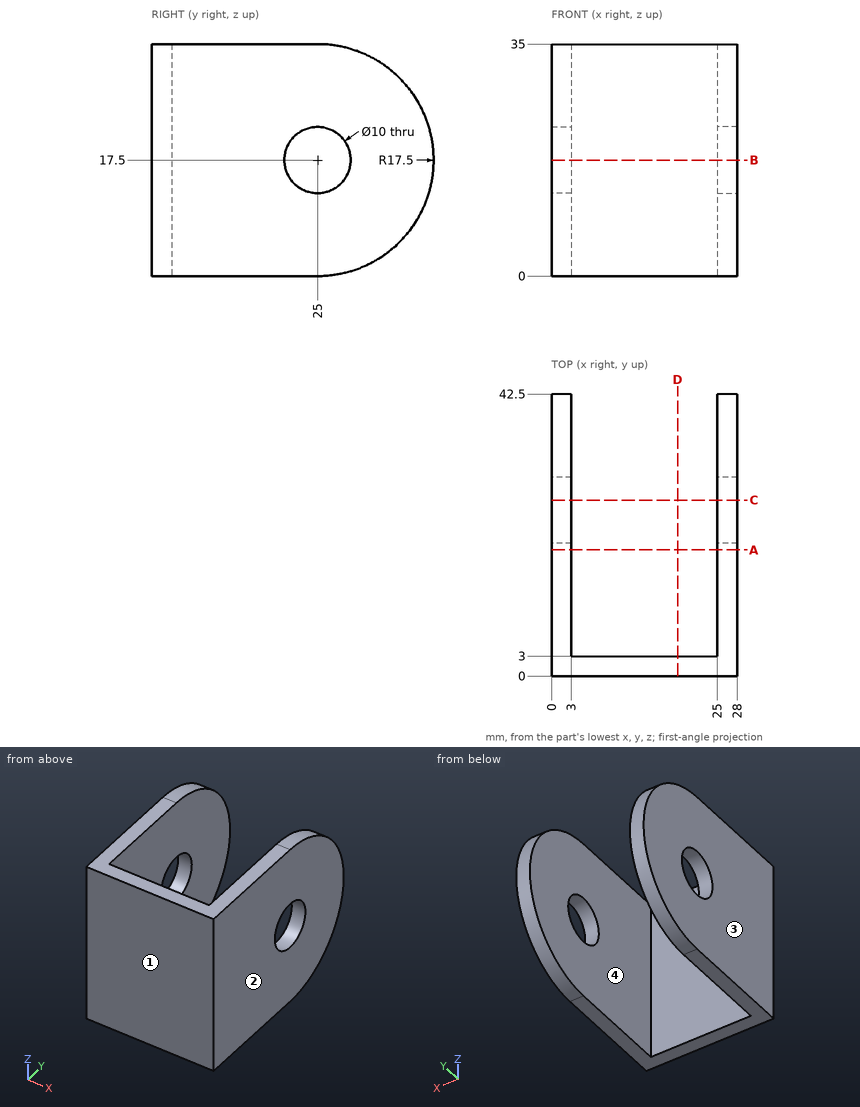
Job drawing, mm, ordinate dimensions from the low corner. One solid piece. Coordinates: 2 decimals unless noted, no trailing zeros. Order: outer loops, then holes, each group sorted by start corner. A loop starts at its lowest first (then second) coordinate and runs counter-clockwise, first axis right, second up. Notation, with made-up numbers: (-13.75, -4.5) -> (34.25, -4.5) arc R8 cw to (34.25, 0.5) -> close; hole circle Ø5 at (-17.75, -31). An arc over 180 degrees is marked (long way). Return JSON: item names as keys, results as strings. Group by question number.
Item 1: Pull direction X, two halves, no side cores. Call the marked faces 1, 2, 3 and 4: pulls with the +X half, pulls with the -X half, needs draft (parallel to the pull), parting line crosses it, or undercut.
Item 2: Wall check: line 1 along X through (y, z) = (31, 33); line 2 along Y through (x, z) = (2.2, 17.5); line 3 along Z through (x, y) = (1.9, 25). Give the ranges that are in metal, low to high. Write a range as [from, to].
Item 3: Saw through at A-A on y = 19. Write the cut outline in (x, z), then the cut area to 3 significant figures.
Item 4: Flat gauge pins, fed straight in: P1, Ø5, axis at x = 10, z = 18.5, coming from the -Y side; P2, Ø11, axis at x = 16.5, z = 17.5, coming from the +Y side. Where does each tip first touch, or does it go through?
Item 5: Saw through at D-D on x = 19. Write the cut outline in (y, z).
Item 6: Saw through at B-B on z = 17.5. Write the cut outline in (x, y).
Item 7: Saw through at C-C on y = 26.5. Write the cut outline in (x, z).
Values found:
{
 "1": {"face 1": "needs draft", "face 2": "pulls with the +X half", "face 3": "pulls with the -X half", "face 4": "undercut"},
 "2": {"line 1": "x = [0, 3], [25, 28]", "line 2": "y = [0, 20], [30, 42.5]", "line 3": "z = [0, 12.5], [22.5, 35]"},
 "3": {"outline": "(0, 0) -> (3, 0) -> (3, 35) -> (0, 35) -> close; (25, 0) -> (28, 0) -> (28, 35) -> (25, 35) -> close", "area": "210 mm2"},
 "4": {"P1": "stops at y = 0", "P2": "stops at y = 3"},
 "5": {"outline": "(0, 0) -> (3, 0) -> (3, 35) -> (0, 35) -> close"},
 "6": {"outline": "(0, 0) -> (28, 0) -> (28, 20) -> (25, 20) -> (25, 3) -> (3, 3) -> (3, 20) -> (0, 20) -> close; (0, 30) -> (3, 30) -> (3, 42.5) -> (0, 42.5) -> close; (25, 30) -> (28, 30) -> (28, 42.5) -> (25, 42.5) -> close"},
 "7": {"outline": "(0, 0.06) -> (3, 0.06) -> (3, 12.73) -> (0, 12.73) -> close; (0, 22.27) -> (3, 22.27) -> (3, 34.94) -> (0, 34.94) -> close; (25, 0.06) -> (28, 0.06) -> (28, 12.73) -> (25, 12.73) -> close; (25, 22.27) -> (28, 22.27) -> (28, 34.94) -> (25, 34.94) -> close"}
}
